Design review of the part built by this model. Coordinates are the model's own, in mm. Face numbers are marked on the shaded views. A direction names the side the tool comes from. Give positions to 0.01 mm unless a question says otherwise; leave off trailing zeros. Order: outer loops, then holes, each group sorted by start corner. A loop starts at its lowest first (then second) coordinate and runs counter-clockwise, first axis right, second up. Notation, with made-up numbers: (-5.5, 43.5) -> (-0.5, 43.5) arc R30 ccw to (-0.5, 75.5) -> close; hole circle Ø2 at (-4.75, 54). An arc over 180 degrees is marked (long way). Return JSON: item names as keys, results as strings.
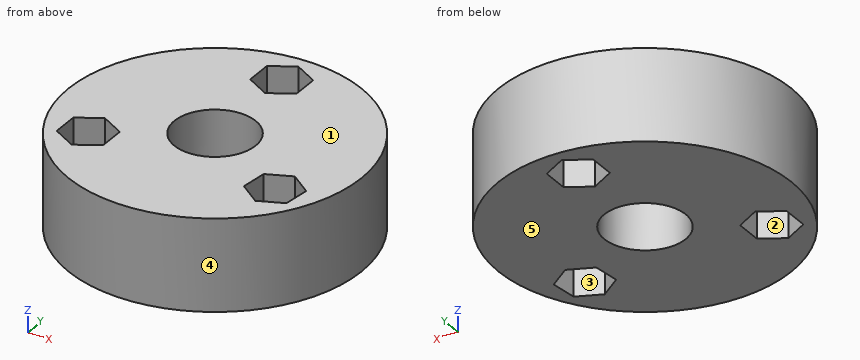
```python
from build123d import *

# Parameters (mm, degrees)
F0_R     = 40
F0_R_2   = 11.1125
F1_DEPTH = 7.5
F2_DEPTH = 25


with BuildPart() as f1:
    # F0 (on Top) → F1 (new body)
    with BuildSketch(Plane.XY):
        Circle(F0_R)
        Polygon((-25.510716, -7.39627), (-19.160716, -11.062445), (-19.160716, -18.394793), (-25.510716, -22.060967), (-31.860716, -18.394793), (-31.860716, -11.062445), align=None, mode=Mode.SUBTRACT)
        Polygon((26.423282, -7.45328), (32.267627, -11.881254), (31.355062, -19.156593), (24.59815, -22.003958), (18.753805, -17.575983), (19.666371, -10.300644), align=None, mode=Mode.SUBTRACT)
        Circle(F0_R_2, mode=Mode.SUBTRACT)
        Polygon((0, 36.789586), (6.35, 33.123412), (6.35, 25.791063), (0, 22.124889), (-6.35, 25.791063), (-6.35, 33.123412), align=None, mode=Mode.SUBTRACT)
    extrude(amount=F1_DEPTH)

    # F0 (on Top) → F2 (join)
    with BuildSketch(Plane.XY):
        Circle(F0_R)
        Polygon((-25.510716, -7.39627), (-19.160716, -11.062445), (-19.160716, -18.394793), (-25.510716, -22.060967), (-31.860716, -18.394793), (-31.860716, -11.062445), align=None, mode=Mode.SUBTRACT)
        Polygon((26.423282, -7.45328), (32.267627, -11.881254), (31.355062, -19.156593), (24.59815, -22.003958), (18.753805, -17.575983), (19.666371, -10.300644), align=None, mode=Mode.SUBTRACT)
        Circle(F0_R_2, mode=Mode.SUBTRACT)
        Polygon((0, 36.789586), (6.35, 33.123412), (6.35, 25.791063), (0, 22.124889), (-6.35, 25.791063), (-6.35, 33.123412), align=None, mode=Mode.SUBTRACT)
    extrude(amount=F2_DEPTH)


solid = f1.part
```
Item 1: Add section A-A (y = 0). Give the boundary of the cut face in (x, z), plus the area to 3 significant figures.
Result set:
{"outline": "(-40, 0) -> (-11.11, 0) -> (-11.11, 25) -> (-40, 25) -> close; (11.11, 0) -> (40, 0) -> (40, 25) -> (11.11, 25) -> close", "area": "1,440 mm^2"}
Item 2: Wall thickness on L1, parallel to Y at x = 0, z = 8.25; L2, parallel to Y at x = -9, z = 13.25; L3, parallel to X at y = 20, z = 1.5: over which ranges is each line inside the solid? List them lowest first. Write a range as [from, to].
Result set:
{"L1": "y = [-40, -11.11], [11.11, 22.12], [36.79, 40]", "L2": "y = [-38.97, -6.52], [6.52, 38.97]", "L3": "x = [-34.64, 34.64]"}
Item 3: Add section B-B (z = 7.5). Give the number of separate pieces and of enclosed holes in the cut face, plus the area to 3 significant figures.
Result set:
{"separate pieces": "1", "enclosed holes": "4", "area": "4,220 mm^2"}
Item 4: Machinability: for the marked faces 1 and 2, which of the approach directions +Z, -Z, +X, -X, +Y, -Y give a long, thin tool a straight path to every point of the face, cutting with its end or side? Answer none if there is none.
Result set:
{"face 1": "+Z, +X, -X, +Y, -Y", "face 2": "+Z, -Z"}
Item 5: Mouldability with a two-part tool opening along X and no side actions: class the marked faces 3, 4 and 5 as released by +X, released by -X, zero draft, split by the parting line, or undercut.
Result set:
{"face 3": "undercut", "face 4": "split by the parting line", "face 5": "zero draft"}
Item 6: Add section C-C (y = -8.5). Give the boundary of the cut face in (x, z), plus the area to 3 significant figures.
Result set:
{"outline": "(-39.09, 0) -> (-27.42, 0) -> (-27.42, 25) -> (-39.09, 25) -> close; (-23.6, 0) -> (-7.16, 0) -> (-7.16, 25) -> (-23.6, 25) -> close; (7.16, 0) -> (23.94, 0) -> (23.94, 25) -> (7.16, 25) -> close; (27.8, 0) -> (39.09, 0) -> (39.09, 25) -> (27.8, 25) -> close", "area": "1,400 mm^2"}
Item 7: For pin 1 (8 mm diameter, centred on y = 31.5, z = 12.5, fed in from +X); pin 2 (2 mm diameter, centred on y = 29.5, z = 9, fed in from -X); pin 3 (10 mm diameter, centred on x = -11, z = 21, fed in from +Y), all flat-tipped, find the tip position at first contact; note any pin that passes through.
Result set:
{"pin 1": "stops at x = 29.05", "pin 2": "stops at x = -28.07", "pin 3": "stops at y = 39.55"}
Item 8: Add section D-D (y = 8.5). Give the boundary of the cut face in (x, z), plus the area to 3 significant figures.
Result set:
{"outline": "(-39.09, 0) -> (-7.16, 0) -> (-7.16, 25) -> (-39.09, 25) -> close; (7.16, 0) -> (39.09, 0) -> (39.09, 25) -> (7.16, 25) -> close", "area": "1,600 mm^2"}
